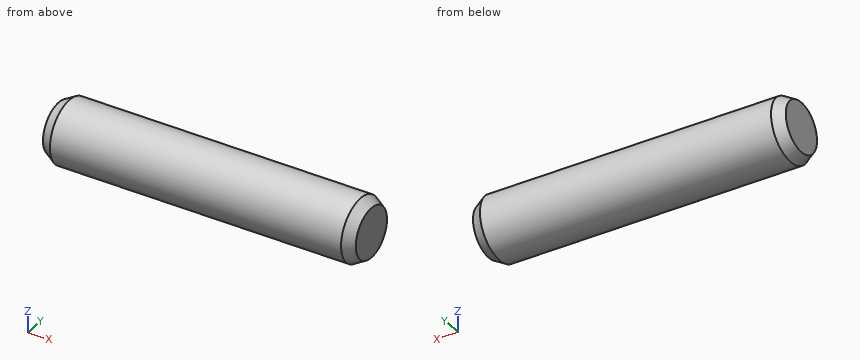
```python
from build123d import *

# Parameters (mm, degrees)
SKETCH4_R           = 5
BOSS_EXTRUDE2_DEPTH = 50
CHAMFER1_SIZE       = 1
CHAMFER1_SIZE2      = 1.732050808
CHAMFER2_SIZE       = 1
CHAMFER2_SIZE2      = 1.732050808


with BuildPart() as part:
    # Sketch4 → Boss-Extrude2 (new body)
    with BuildSketch(Plane(origin=(0, 0, 0), x_dir=(0, 0, -1), z_dir=(1, 0, 0))):
        Circle(SKETCH4_R)
    extrude(amount=BOSS_EXTRUDE2_DEPTH)

    # Chamfer1
    chamfer1_edges = [part.edges().sort_by_distance(p)[0] for p in [
        (0, 0, 5),
    ]]
    chamfer1_side = [part.faces().sort_by_distance(p)[0] for p in [
        (0, 0, 0),
    ]]
    chamfer(chamfer1_edges, length=CHAMFER1_SIZE, length2=CHAMFER1_SIZE2, reference=chamfer1_side[0])

    # Chamfer2
    chamfer2_edges = [part.edges().sort_by_distance(p)[0] for p in [
        (50, 0, 5),
    ]]
    chamfer2_side = [part.faces().sort_by_distance(p)[0] for p in [
        (50, 0, 0),
    ]]
    chamfer(chamfer2_edges, length=CHAMFER2_SIZE, length2=CHAMFER2_SIZE2, reference=chamfer2_side[0])


solid = part.part
```
CAD build for the part. Positions are in the model's coordinates, mm. Round coordinates to 2 decimals unless told otherwise and drop trailing zeros. Loops run counter-clockwise (first coordinate to the right, second up) from the corner with the lowest first, then second, coordinate; pieces in that order, holes last. Notation, with made-up numbers: M -33,29.5 L -8,29.5 A33 cw -8,67.5 Z; hole C 27.5,4 d8. An arc over 180 degrees is marked long. Return JSON: item names as keys, results as strings. Group by question number.
(1) Wall check: probe 1 along Z at (x, y) = (3.5, -3); probe 2 along Z at (x, y) = (8, -0.25). Give the ranges that are in metal, low to high. Write a range as [from, to].
(2) Drop flat-ended pins along their axis: P1, Ø1.5, axis at x = 6, z = -3, coming from the -Y side; P2, Ø3, axis at x = 28, y = 3.5, coming from the -Z side; P3, Ø1.5, axis at x = 13.5, z = 2.5, coming from the +Y side. Give the stop position or say it passes through.
(3) Saw through at A-A, the plane x = 16.5. List the corners of the cut face in (y, z).
Answer list:
{
 "1": {"probe 1": "[-4, 4]", "probe 2": "[-4.99, 4.99]"},
 "2": {"P1": "y = -4.47", "P2": "z = -4.58", "P3": "y = 4.68"},
 "3": {"outline": "C 0,0 d10"}
}
